from build123d import *

# Parameters (mm, degrees)
SKETCH_1_R      = 1.25
SKETCH_1_R_2    = 1.5
EXTRUDE_1_DEPTH = 4
FILLET_1_R      = 3


with BuildPart() as part:
    # 草图1 → 凸台-拉伸1 (new body)
    with BuildSketch(Plane.XY):
        with BuildLine():
            Line((-6.635089387, 15.274909239), (16.252937679, 7.354644413))
            Line((16.252937679, 7.354644413), (16.252937679, 32.645355587))
            Line((16.252937679, 32.645355587), (-6.635089387, 24.725090761))
            ThreePointArc((-6.635089387, 24.725090761), (-10, 20), (-6.635089387, 15.274909239))
        make_face()
        with Locations((-5, 20)):
            Circle(SKETCH_1_R, mode=Mode.SUBTRACT)
        with Locations((10, 26)):
            Circle(SKETCH_1_R_2, mode=Mode.SUBTRACT)
        with Locations((10, 14)):
            Circle(SKETCH_1_R_2, mode=Mode.SUBTRACT)
    extrude(amount=EXTRUDE_1_DEPTH)

    # 圆角1
    fillet_1_edges = [part.edges().sort_by_distance(p)[0] for p in [
        (16.252937679, 32.645355587, 2),
        (16.252937679, 7.354644413, 2),
    ]]
    fillet(fillet_1_edges, radius=FILLET_1_R)


solid = part.part
Could you check a few things on this model? Use its own coordinates, in mm. Round coordinates to 2 decimals unless told otherwise and drop trailing zeros. Order: outer loops, then holes, each group sorted by start corner. A loop starts at its lowest first (then second) coordinate and runs counter-clockwise, first axis right, second up.
(1) Imagine slicing it at C-C (x = -5.25). Write out the boundary of the cut face in (y, z), plus the area to 3 significant figures.
Response values:
outline: (14.8, 0) - (18.78, 0) - (18.78, 4) - (14.8, 4) - close; (21.22, 0) - (25.2, 0) - (25.2, 4) - (21.22, 4) - close
area: 31.8 mm2
(2) Imagine slicing it at A-A (z = 0.3). Write out the boundary of the cut face in (x, y), plus the area to 3 significant figures.
Response values:
outline: (-6.64, 15.27) - (12.27, 8.73) arc R3 ccw to (16.25, 11.57) - (16.25, 28.43) arc R3 ccw to (12.27, 31.27) - (-6.64, 24.73) arc R5 ccw to start; hole circle Ø2.5 at (-5, 20); hole circle Ø3 at (10, 14); hole circle Ø3 at (10, 26)
area: 394 mm2
(3) Please list where these lines run through material, in increasing order: line 1 along Y through (x, z) = (10, 2.85); line 2 along Y through (x, z) = (9.75, 3.1); line 3 along Y through (x, z) = (-5, 1.4).
Response values:
line 1: y = 9.52 to 12.5, 15.5 to 24.5, 27.5 to 30.48
line 2: y = 9.6 to 12.52, 15.48 to 24.52, 27.48 to 30.4
line 3: y = 14.71 to 18.75, 21.25 to 25.29
(4) I'm going to push flat-ended pins straight in: pin 1 (2 mm diameter, centred on x = -5, z = 2.5, fed in from +Y); pin 2 (2 mm diameter, centred on x = -5, y = 20, fed in from +Z); pin 3 (2 mm diameter, centred on x = -1.5, z = 3, fed in from +Y); pin 4 (2 mm diameter, centred on x = -3, z = 1, fed in from +Y). Where does each tip first touch, or does it pass through?
Response values:
pin 1: stops at y = 25.64
pin 2: passes through
pin 3: stops at y = 26.85
pin 4: stops at y = 26.33
(5) Imagine slicing it at B-B (y = 20). Write out the boundary of the cut face in (x, z), plus the area to 3 significant figures.
Response values:
outline: (-10, 0) - (-6.25, 0) - (-6.25, 4) - (-10, 4) - close; (-3.75, 0) - (16.25, 0) - (16.25, 4) - (-3.75, 4) - close
area: 95.0 mm2
(6) Imagine slicing it at D-D (x = 10). Write out the boundary of the cut face in (y, z), plus the area to 3 significant figures.
Response values:
outline: (9.52, 0) - (12.5, 0) - (12.5, 4) - (9.52, 4) - close; (15.5, 0) - (24.5, 0) - (24.5, 4) - (15.5, 4) - close; (27.5, 0) - (30.48, 0) - (30.48, 4) - (27.5, 4) - close
area: 59.9 mm2
(7) If we mould it in two halves opening along X, with no side actions, what happens to faces 1 (the flat face through (2.95, 28.04, 1.97)), 2 (the cylindrical face through (15.03, 30.85, 2.03)), 3 (the cylindrical face through (8.5, 14.07, 1.97))? For each: released by +X, released by -X, zero draft, split by the parting line, or undercut.
Response values:
face 1: released by -X
face 2: split by the parting line
face 3: undercut
